Autodesk Inventor part; units mm, degrees
ref_plane "YZ Plane" through (0, 0, 0) normal (1, 0, 0) x (0, 1, 0)
ref_plane "XZ Plane" through (0, 0, 0) normal (0, 1, 0) x (-1, 0, 0)
ref_plane "XY Plane" through (0, 0, 0) normal (0, 0, 1) x (1, 0, 0)
sketch "Sketch1" plane through (0, 0, 0) normal (0, 0, 1) x (1, 0, 0)
  line L0 (-165.1, 0) -> (165.1, 0) construction
  line L1 (-215.9, -25.4) -> (-165.1, -25.4)
  line L2 (-165.1, -25.4) -> (-165.1, 25.4)
  line L3 (-165.1, 25.4) -> (-215.9, 25.4)
  line L4 (-215.9, 25.4) -> (-215.9, -25.4)
  line L5 (-215.9, -25.4) -> (-165.1, 25.4) construction
  line L6 (-165.1, -25.4) -> (-215.9, 25.4) construction
  line L7 (215.9, -25.4) -> (165.1, -25.4)
  line L8 (165.1, -25.4) -> (165.1, 25.4)
  line L9 (165.1, 25.4) -> (215.9, 25.4)
  line L10 (215.9, 25.4) -> (215.9, -25.4)
  line L11 (215.9, -25.4) -> (165.1, 25.4) construction
  line L12 (165.1, -25.4) -> (215.9, 25.4) construction
  line L13 (-168.275, 22.225) -> (-168.275, -22.225)
  line L14 (-168.275, -22.225) -> (-212.725, -22.225)
  line L15 (-212.725, -22.225) -> (-212.725, 22.225)
  line L16 (-212.725, 22.225) -> (-168.275, 22.225)
  line L17 (212.725, -22.225) -> (168.275, -22.225)
  line L18 (168.275, -22.225) -> (168.275, 22.225)
  line L19 (168.275, 22.225) -> (212.725, 22.225)
  line L20 (212.725, 22.225) -> (212.725, -22.225)
  point P0 (0, 0)
  point P1 (0, 0)
  point P2 (-190.5, 0)
  point P3 (190.5, 0)
  dimension "d0" = 330.2
  dimension "d1" = 50.8
  dimension "d2" = 3.175
  dimension "d3" = 3.175
extrude "Extrusion1" add sketch "Sketch1" along normal blind 209.55
sketch "Sketch2" plane through (215.9, -25.4, 0) normal (1, 0, 0) x (0, 0, -1)
  line L0 (0, 25.4) -> (-209.55, 25.4) construction
  line L1 (-209.55, 3.175) -> (-209.55, 47.625) construction
  circle A0 centre (-190.5, 25.4) radius 15.875
  circle A1 centre (-190.5, 25.4) radius 12.7
  dimension "d6" = 31.75
  dimension "d7" = 19.05
  dimension "d8" = 3.175
extrude "Extrusion2" add sketch "Sketch2" against normal up to surface (431.8 mm away)
sketch "Sketch3" plane through (-215.9, 25.4, 0) normal (0, 1, 0) x (1, 0, 0)
  line L0 (431.8, 0) -> (0, 0)
  line L1 (0, 0) -> (0, 50.8)
  line L2 (0, 50.8) -> (431.8, 50.8)
  line L3 (431.8, 50.8) -> (431.8, 0)
  point P0 (215.9, 0)
  point P1 (215.9, 0)
  dimension "d11" = 431.8
  dimension "d12" = 50.8
extrude "Extrusion3" add sketch "Sketch3" against normal blind 2143.125
properties part number "rung" material "Aluminum 6061"
Input: part model. Units: mm. Frame: model coordinates. A direction names the side the tool comes from. Coordinates: 2 decimals unless noted, no trailing zeros. Write each loop counter-clockwise with the first axis right and the second up, starting at its lowest first coordinate (ties: lowest second). Pieces come first, ordered by that corner, then holes. Notation, with made-up numbers: M -28.75,5 L 29.25,5 A25 cw 29.25,31 Z; hole C -0.75,-27 d6. An arc over 180 degrees is marked long. Use one line per item in the form item = value.
Q1. Draft query along X for faces 1 (the face through (-190, -22.225, 103)), 2 (the face through (-3, -1031, -50.8)), 3 (the face through (-215.9, -882, -16)), 4 (the face through (168.275, 0, 103)). Return one class per face: released by +X, released by -X, zero draft, split by the parting line, or undercut.
Answer below:
face_1 = undercut
face_2 = zero draft
face_3 = released by -X
face_4 = undercut
Q2. First-contact query: pin 1 (22 mm diameter, centred on x = 186, y = -3.5, fed in from +Z) (3 decimals); pin 2 (1.5 mm diameter, centred on x = -111, y = -881.5, fed in from +Z); pin 3 (15 mm diameter, centred on x = -181.5, z = 90.5, fed in from -Y). Flat tips, straight axial feed; report the tip coordinate or a pass-through.
Answer below:
pin_1 = 206.375
pin_2 = 0
pin_3 = -25.4
Q3. Material intervals for probe 1 along Y at (x, z) = (183, 190) (3 decimals); probe 2 along Y at (x, z) = (6, 190); probe 3 along Y at (x, z) = (185, 181) (3 decimals), sorted ascending. Write a range as from..to.
Answer below:
probe_1 = -25.4..-22.225, -15.867..-12.69, 12.69..15.867, 22.225..25.4
probe_2 = -15.87..-12.69, 12.69..15.87
probe_3 = -25.4..-22.225, -12.719..-8.429, 8.429..12.719, 22.225..25.4
Q4. Section C-C (y = -1772). Return loops of the section in (x, z).
Answer below:
outline = M -215.9,-50.8 L 215.9,-50.8 L 215.9,0 L -215.9,0 Z
Q5. Section A-A (z = 92). Return loops of the section in (x, y) (3 decimals), plus the area to 3 significant figures.
Answer below:
outline = M -215.9,-25.4 L -165.1,-25.4 L -165.1,25.4 L -215.9,25.4 Z; M 165.1,-25.4 L 215.9,-25.4 L 215.9,25.4 L 165.1,25.4 Z; hole M -212.725,-22.225 L -168.275,-22.225 L -168.275,22.225 L -212.725,22.225 Z; hole M 168.275,-22.225 L 212.725,-22.225 L 212.725,22.225 L 168.275,22.225 Z
area = 1,210 mm²
Q6. Set-up query: faces 5 (the face through (-191, -25.4, 103)), 6 (the face through (190, 22.225, 103)), 7 (the face through (-190, 0, 0)). Return all of +Z, -Z, +X, -X, +Y, -Y with unobstructed straight access to the full face (end or side cutting, diameter ignored); none if empty.
Answer below:
face_5 = +Z, +X, -X, -Y
face_6 = +Z
face_7 = none
Q7. Section B-B (x = -139). Return loops of the section in (y, z) (3 decimals), plus the area to 3 significant figures.
Answer below:
outline = M -2117.725,-50.8 L 25.4,-50.8 L 25.4,0 L -2117.725,0 Z; C 0,190.5 d31.75; hole C 0,190.5 d25.4
area = 109,000 mm²
